Work out the finished part from the listing and answer in its coordinate system (mm). Face numbers are marked on the shaded views. A direction names the side the tool comes from. Coordinates: 2 decimals unless noted, no trailing zeros. Order: outer loops, then holes, each group sorted by start corner. A loop starts at its lowest first (then second) coordinate and runs counter-clockwise, first axis right, second up. Notation, with made-up numbers: (-32.5, -39) -> (-3.5, -39) arc R10 ccw to (-3.5, -35) -> close; hole circle Ø2 at (43.25, -14.75). An arc over 180 degrees is marked (long way). Write item = value, one per line. Start each with the question number.
Q1. The part is cut by section C-C, the plane z = -6. Determine the outline of the cut face in (x, y), plus the area to 3 significant figures.
Q2. The part is cut by section D-D, the plane y = 2.5. Count the separate pieces of the cut face and the enclosed holes in it, plus the area to 3 significant figures.
Q3. The part is cut by section B-B, the plane y = -3. Determine the outline of the cut face in (x, z).
Q4. The part is cut by section A-A, the plane z = -31.75. Determine the outline of the cut face in (x, y), plus the area to 3 significant figures.
Q5. For a pull along X with two mould halves and no side action, classify the marked faces 1, 2 and 3 as +X half, -X half, draft (parallel to the pull), parting line (faces both ways), or undercut.
Q6. Flat-ended cylindrical pins translate along their axes: pin 1 (4 mm diameter, centred on x = -20.64, z = -22.22, fed in from +Y); pin 2 (3.5 mm diameter, centred on x = 37, y = -0.5, fed in from -Z); pin 3 (12 mm diameter, centred on x = -8.5, z = -10.5, fed in from +Y); pin 4 (6.5 mm diameter, centred on x = 20.64, z = -22.22, fed in from -Y). Find the tip coordinate at first contact, or state that the pin passes through.
Q7. Straight lines are drawn through the part: L1, parallel to X at y = 2.75, z = -31.75; L2, parallel to X at y = 5, z = 31.75; L3, parallel to X at y = -6.5, z = 23.5. For each, find the intervals that lie inside material, in ascending order. Write a range as from..to.
Q8. Which of the six approach directions +Z, -Z, +X, -X, +Y, -Y give full straight-line access (tool end or side, diameter ignored) to the marked faces 4, 5 and 6?
```python
from build123d import *

# Parameters (mm, degrees)
SKETCH_2_W               = 62
SKETCH_2_H               = 84
EXTRUDE_1_DEPTH          = 7
CUT_EXTRUDE_1_DEPTH      = 53.668776329
CUT_EXTRUDE_1_DEPTH_BACK = 53.668776329
SKETCH_4_R               = 2.54
FILLET_1_R               = 5
FILLET_4_R               = 5
EXTRUDE_2_DEPTH          = 8
EXTRUDE_2_DEPTH_BACK     = 9
SKETCH_5_W               = 11
SKETCH_5_H               = 40
SKETCH_11_W              = 10
SKETCH_11_H              = 9
EXTRUDE_3_DEPTH          = 9


with BuildPart() as part:
    # 스케치2 → 보스-돌출1 (new body)
    with BuildSketch(Plane(origin=(0, 0, 0), x_dir=(1, 0, 0), z_dir=(0, 1, 0))):
        Rectangle(SKETCH_2_W, SKETCH_2_H)
    extrude(amount=EXTRUDE_1_DEPTH)

    # 스케치4 → 컷-돌출1 (cut, two sides: drawn at the far end of the back side and taken through both)
    with BuildSketch(Plane.XZ.offset(-CUT_EXTRUDE_1_DEPTH_BACK)):
        with Locations(Location((20.6375, 31.75, 0), (0, 0, 270))):
            Circle(SKETCH_4_R)
        with Locations(Location((20.6375, -22.225, 0), (0, 0, 270))):
            Circle(SKETCH_4_R)
        with Locations(Location((20.6375, -31.75, 0), (0, 0, 270))):
            Circle(SKETCH_4_R)
        with Locations(Location((-20.6375, -31.75, 0), (0, 0, 270))):
            Circle(SKETCH_4_R)
        with Locations(Location((-20.6375, -22.225, 0), (0, 0, 270))):
            Circle(SKETCH_4_R)
        with Locations(Location((-20.6375, 31.75, 0), (0, 0, 270))):
            Circle(SKETCH_4_R)
    extrude(amount=CUT_EXTRUDE_1_DEPTH + CUT_EXTRUDE_1_DEPTH_BACK, mode=Mode.SUBTRACT)

    # 필렛1
    fillet_1_edges = [part.edges().sort_by_distance(p)[0] for p in [
        (-31, 3.5, -42),
        (31, 3.5, -42),
    ]]
    fillet(fillet_1_edges, radius=FILLET_1_R)

    # 필렛4
    fillet_4_edges = [part.edges().sort_by_distance(p)[0] for p in [
        (31, 3.5, 42),
        (-31, 3.5, 42),
    ]]
    fillet(fillet_4_edges, radius=FILLET_4_R)

    # 스케치5 → 보스-돌출2 (add, two sides: drawn at the far end of the back side and taken through both)
    with BuildSketch(Plane.XZ.offset(-EXTRUDE_2_DEPTH_BACK)):
        with Locations((-34.5, 7)):
            Rectangle(SKETCH_5_W, SKETCH_5_H)
        with Locations((34.5, 7)):
            Rectangle(SKETCH_5_W, SKETCH_5_H)
    extrude(amount=EXTRUDE_2_DEPTH + EXTRUDE_2_DEPTH_BACK)

    # 스케치11 → 보스-돌출3 (add)
    with BuildSketch(Plane(origin=(31, 0, 0), x_dir=(0, 0, -1), z_dir=(1, 0, 0))):
        with Locations((-32, 4.5)):
            Rectangle(SKETCH_11_W, SKETCH_11_H)
    extrude(amount=EXTRUDE_3_DEPTH)


solid = part.part
```
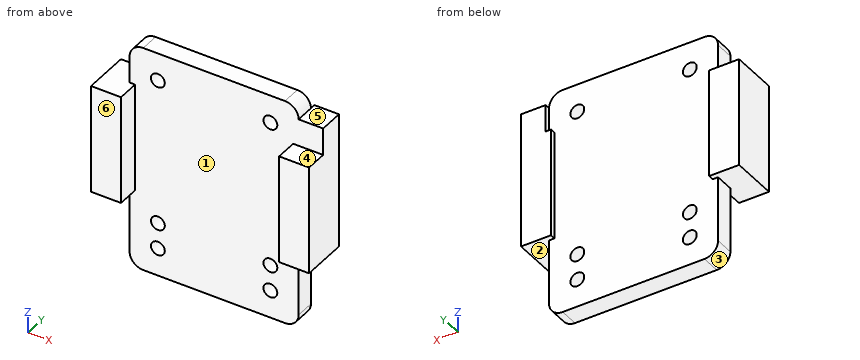
Model answer:
q1.outline = (-40, -8) -> (-29, -8) -> (-29, 0) -> (29, 0) -> (29, -8) -> (40, -8) -> (40, 9) -> (29, 9) -> (29, 7) -> (-29, 7) -> (-29, 9) -> (-40, 9) -> close
q1.area = 780 mm2
q2.separate_pieces = 1
q2.enclosed_holes = 6
q2.area = 5,870 mm2
q3.outline = (-40, -13) -> (-29, -13) -> (-29, 27) -> (-40, 27) -> close; (29, -13) -> (40, -13) -> (40, 27) -> (29, 27) -> close
q4.outline = (-31, 0) -> (-23.18, 0) -> (-23.18, 7) -> (-31, 7) -> close; (-18.1, 0) -> (18.1, 0) -> (18.1, 7) -> (-18.1, 7) -> close; (23.18, 0) -> (31, 0) -> (31, 7) -> (23.18, 7) -> close
q4.area = 363 mm2
q5.face_1 = undercut
q5.face_2 = draft
q5.face_3 = -X half
q6.pin_1 = through
q6.pin_2 = -13
q6.pin_3 = 7
q6.pin_4 = 0
q7.L1 = -31..-23.18, -18.1..18.1, 23.18..31
q7.L2 = -31..-23.18, -18.1..18.1, 23.18..40
q7.L3 = -40..-29, 29..40
q8.face_4 = +Z, +X, -X, -Y
q8.face_5 = +Z, +X, +Y, -Y
q8.face_6 = +Z, -Z, +X, -X, -Y
